Work out the finished part from the listing and answer in its coordinate system (mm). Coordinates: 2 decimals unless noted, no trailing zeros. Order: outer loops, then holes, each group sorted by start corner. A loop starts at its lowest first (then second) coordinate and runs counter-clockwise, first axis right, second up.
1. The part is cut by section B-B, the plane x = 98. Give the vertices of the cut face in (y, z), then the cut area to 3 significant figures.
2. The part is cut by section C-C, the plane y = -46. Give the vertices of the cut face in (x, z), then the cut area to 3 significant figures.
3. Find the intervals of material crossed by probe 1 along X at (y, z) = (-150, 0.95); probe 2 along Y at (x, z) = (0, 0.75); probe 3 along Y at (x, z) = (14.5, 0.55), in increasing order.
4. The part is cut by section D-D, the plane x = 161.5. Give the vertices of the cut face in (y, z).
5. The part is cut by section A-A, the plane z = 0.8. Count the separate pieces of the cut face and the enclosed holes in it, then the cut area to 3 significant figures.
6. Flat-ended cylindrical pins translate along their axes: pin 1 Ø4.5 at (x, y) = (-135.8, 4) entering from -Z; pin 2 Ø2 at (x, z) = (4.5, 1) entering from -Y; pin 3 Ø1.5 at (x, z) = (81.5, 2.5) entering from -Y; pin 4 Ø2 at (x, z) = (115, 1) entering from -Y. Find the tip coordinate at first contact, or state that the pin passes through.
Autodesk Inventor part; units mm, degrees
ref_plane "YZ Plane" through (0, 0, 0) normal (1, 0, 0) x (0, 1, 0)
ref_plane "XZ Plane" through (0, 0, 0) normal (0, 1, 0) x (-1, 0, 0)
ref_plane "XY Plane" through (0, 0, 0) normal (0, 0, 1) x (1, 0, 0)
sketch "Sketch1" plane through (0, 0, 0) normal (0, 0, 1) x (1, 0, 0)
  line L0 (11.9, 0) -> (6, 0) construction
  line L1 (6, 4) -> (11.9, 4) construction
  line L2 (-150.8, -316.8297) -> (-150.8003, 183.1703) construction
  line L3 (210, 14) -> (-150.8001, 14)
  line L4 (-150.8001, 14) -> (-150.8001, -160)
  line L5 (-150.8001, -160) -> (-120.8001, -160)
  line L6 (210, -7.5086) -> (210, 14)
  line L7 (-120.8, -316.8296) -> (-120.8003, 183.1704) construction
  line L8 (-120.8001, -160) -> (210, -7.5086)
  line L9 (425, -160) -> (0, -160)
  line L10 (6, 4) -> (6, 0)
  line L11 (11.9, 0) -> (11.9, 4)
  dimension "d0" = 10
extrude "Extrusion1" add sketch "Sketch1" along normal blind 4
fillet "Fillet1" radius 2 5 edges at (210, 14, 2) (210, -7.5086, 2) (-150.8001, 14, 2) (-150.8001, -160, 2) (-120.8001, -160, 2)
sketch "Sketch2" plane through (0, 0, 4) normal (0, 0, 1) x (1, 0, 0)
  point P0 (0, 0)
sketch "Sketch3" plane through (0, 0, 4) normal (0, 0, 1) x (1, 0, 0)
  line L0 (200, 0) -> (200, 4)
  line L1 (200, 4) -> (199.5, 4)
  line L2 (194.5, 4) -> (199.5, 4)
  line L3 (194.5, 4) -> (194, 4)
  line L4 (194, 0) -> (194, 4)
  line L5 (194, 0) -> (194.5, 0)
  line L6 (199.5, 0) -> (194.5, 0)
  line L7 (199.5, 0) -> (200, 0)
  line L8 (200.2, 4.2) -> (200.2, -0.2)
  line L9 (200.2, -0.2) -> (199.5, -0.2)
  line L10 (199.5, -0.2) -> (194.5, -0.2)
  line L11 (194.5, -0.2) -> (193.8, -0.2)
  line L12 (193.8, -0.2) -> (193.8, 4.2)
  line L13 (193.8, 4.2) -> (194.5, 4.2)
  line L14 (194.5, 4.2) -> (199.5, 4.2)
  line L15 (199.5, 4.2) -> (200.2, 4.2)
  line L16 (178.3, 0) -> (173.3, 0)
  line L17 (178.3, 0) -> (178.8, 0)
  line L18 (178.8, 0) -> (178.8, 4)
  arc A0 (-121.2388, -160) -> (-120.4016, -159.8163) centre (-121.2388, -158) ccw
  line L19 (-120.4016, -159.8163) -> (208.8373, -8.0446)
  arc A1 (208.8373, -8.0446) -> (210, -6.2283) centre (208, -6.2283) ccw
  line L20 (210, -6.2283) -> (210, 12)
  arc A2 (210, 12) -> (208, 14) centre (208, 12) ccw
  line L21 (208, 14) -> (-148.8001, 14)
  arc A3 (-148.8001, 14) -> (-150.8001, 12) centre (-148.8001, 12) ccw
  line L22 (-150.8001, 12) -> (-150.8001, -158)
  arc A4 (-150.8001, -158) -> (-148.8001, -160) centre (-148.8001, -158) ccw
  line L23 (-148.8001, -160) -> (-121.2388, -160)
  line L24 (178.8, 4) -> (178.3, 4)
  line L25 (173.3, 4) -> (178.3, 4)
  line L26 (173.3, 4) -> (172.8, 4)
  line L27 (172.8, 0) -> (172.8, 4)
  line L28 (172.8, 0) -> (173.3, 0)
  line L29 (21.7, 4) -> (26.7, 4)
  line L30 (27.2, 4) -> (26.7, 4)
  line L31 (27.2, 0) -> (27.2, 4)
  line L32 (26.7, 0) -> (27.2, 0)
  line L33 (26.7, 0) -> (21.7, 0)
  line L34 (21.2, 0) -> (21.7, 0)
  line L35 (21.2, 0) -> (21.2, 4)
  line L36 (21.7, 4) -> (21.2, 4)
  line L37 (6, 0) -> (6, 4)
  line L38 (0, 0) -> (0, 4)
  line L39 (5.5, 0) -> (0.5, 0)
  line L40 (0.5, 4) -> (5.5, 4)
  line L41 (6, 4) -> (5.5, 4)
  line L42 (5.5, 0) -> (6, 0)
  line L43 (0, 0) -> (0.5, 0)
  line L44 (0.5, 4) -> (0, 4)
  line L45 (11.9, 4) -> (15.3, 4)
  line L46 (11.9, 4) -> (11.9, 0)
  line L47 (15.3, 0) -> (11.9, 0)
  line L48 (15.3, 4) -> (15.3, 0)
  line L49 (184.7, 4) -> (188.1, 4)
  line L50 (184.7, 4) -> (184.7, 0)
  line L51 (188.1, 0) -> (184.7, 0)
  line L52 (188.1, 4) -> (188.1, 0)
  line L53 (179, 4.2) -> (179, -0.2)
  line L54 (179, -0.2) -> (178.3, -0.2)
  line L55 (178.3, -0.2) -> (173.3, -0.2)
  line L56 (173.3, -0.2) -> (172.6, -0.2)
  line L57 (172.6, -0.2) -> (172.6, 4.2)
  line L58 (172.6, 4.2) -> (173.3, 4.2)
  line L59 (173.3, 4.2) -> (178.3, 4.2)
  line L60 (178.3, 4.2) -> (179, 4.2)
  line L61 (21.7, -0.2) -> (26.7, -0.2)
  line L62 (26.7, -0.2) -> (27.4, -0.2)
  line L63 (27.4, -0.2) -> (27.4, 4.2)
  line L64 (27.4, 4.2) -> (26.7, 4.2)
  line L65 (26.7, 4.2) -> (21.7, 4.2)
  line L66 (21.7, 4.2) -> (21, 4.2)
  line L67 (21, 4.2) -> (21, -0.2)
  line L68 (21, -0.2) -> (21.7, -0.2)
  line L69 (-0.2, 4.2) -> (-0.2, -0.2)
  line L70 (-0.2, -0.2) -> (0.5, -0.2)
  line L71 (0.5, -0.2) -> (5.5, -0.2)
  line L72 (5.5, -0.2) -> (6.2, -0.2)
  line L73 (6.2, -0.2) -> (6.2, 4.2)
  line L74 (6.2, 4.2) -> (5.5, 4.2)
  line L75 (5.5, 4.2) -> (0.5, 4.2)
  line L76 (0.5, 4.2) -> (-0.2, 4.2)
  circle A5 centre (13.6, 2) radius 1.6
  circle A6 centre (186.4, 2) radius 1.6
  point P0 (0, 0)
  dimension "d5" = 0.2
  dimension "d6" = 0.2
  dimension "d7" = 0.2
  dimension "d8" = 0.2
  dimension "d9" = 3.2
  dimension "d10" = 3.2
extrude "Extrusion2" cut sketch "Sketch3" against normal blind 4 contours L7 L6 L5 L4 L3 L2 L1 L0 | L8 L9 L10 L11 L12 L13 L14 L15 | L16 L28 L27 L26 L25 L24 L18 L17 | L29 L30 L31 L32 L33 L34 L35 L36 | L42 L39 L43 L38 L44 L40 L41 L37 | L53 L54 L55 L56 L57 L58 L59 L60 | L68 L67 L66 L65 L64 L63 L62 L61 | L76 L75 L74 L73 L72 L71 L70 L69 | A5 | A6
sketch "Sketch4" plane through (0, 0, 4) normal (0, 0, 1) x (1, 0, 0)
  line L0 (-139.9, -316.8296) -> (-139.9003, 183.1704) construction
  line L1 (-131.7, -316.8296) -> (-139.9, -316.8296) construction
  line L2 (-131.7, -316.8296) -> (-131.7003, 183.1704) construction
  line L3 (-139.9003, 183.1704) -> (-131.7003, 183.1704) construction
  line L4 (-131.7002, 4) -> (-139.9001, 4) construction
  line L5 (-139.9001, 4) -> (-139.9001, -150) construction
  line L6 (-139.9001, -150) -> (-131.7002, -150) construction
  line L7 (-131.7002, -150) -> (-131.7002, 4) construction
  line L8 (208, 14) -> (-148.8001, 14)
  line L9 (-148.8001, -160) -> (-121.2388, -160)
  circle A0 centre (-135.8001, 4) radius 2.5
  circle A1 centre (-135.8001, -150) radius 2.5
  point P0 (0, 0)
  dimension "d13" = 10
  dimension "d14" = 10
  dimension "d15" = 5
  dimension "d16" = 5
extrude "Extrusion3" cut sketch "Sketch4" against normal blind 4
sketch "Sketch5" plane through (0, 0, 0) normal (0, 0, -1) x (-1, 0, 0)
  line L0 (-131.75, 4) -> (-131.75, 0)
  line L1 (-68.25, 0) -> (-68.25, 4)
  line L2 (-131.75, 0) -> (-68.25, 0)
  line L3 (-68.25, 0) -> (-68.25, 4)
  line L4 (-68.25, 4) -> (-131.75, 4)
  line L5 (-131.75, 4) -> (-131.75, 0)
  line L6 (-131.95, 4.2) -> (-68.05, 4.2)
  line L7 (-68.05, 4.2) -> (-68.05, -0.2)
  line L8 (-68.05, -0.2) -> (-131.95, -0.2)
  line L9 (-131.95, -0.2) -> (-131.95, 4.2)
  point P0 (0, 0)
  dimension "d19" = 0.2
extrude "Extrusion4" cut sketch "Sketch5" against normal blind 25.4 contours L4 L1 L2 L0 | L6 L7 L8 L9
properties part number "Projector mount side"
Geometry says:
1. outline: (-59.14, 0) - (-0.2, 0) - (-0.2, 4) - (-59.14, 4) - close; (4.2, 0) - (14, 0) - (14, 4) - (4.2, 4) - close
1. area: 275 mm2
2. outline: (-150.8, 0) - (126.5, 0) - (126.5, 4) - (-150.8, 4) - close
2. area: 1,110 mm2
3. probe 1: x = -150.8 to -138.3, -133.3 to -99.11
3. probe 2: y = -104.31 to -0.2, 4.2 to 14
3. probe 3: y = -97.63 to 0.68, 3.32 to 14
4. outline: (-29.87, 0) - (14, 0) - (14, 4) - (-29.87, 4) - close
5. separate pieces: 1
5. enclosed holes: 9
5. area: 37,100 mm2
6. pin 1: passes through
6. pin 2: stops at y = -102.7
6. pin 3: stops at y = -67.09
6. pin 4: stops at y = -51.76
